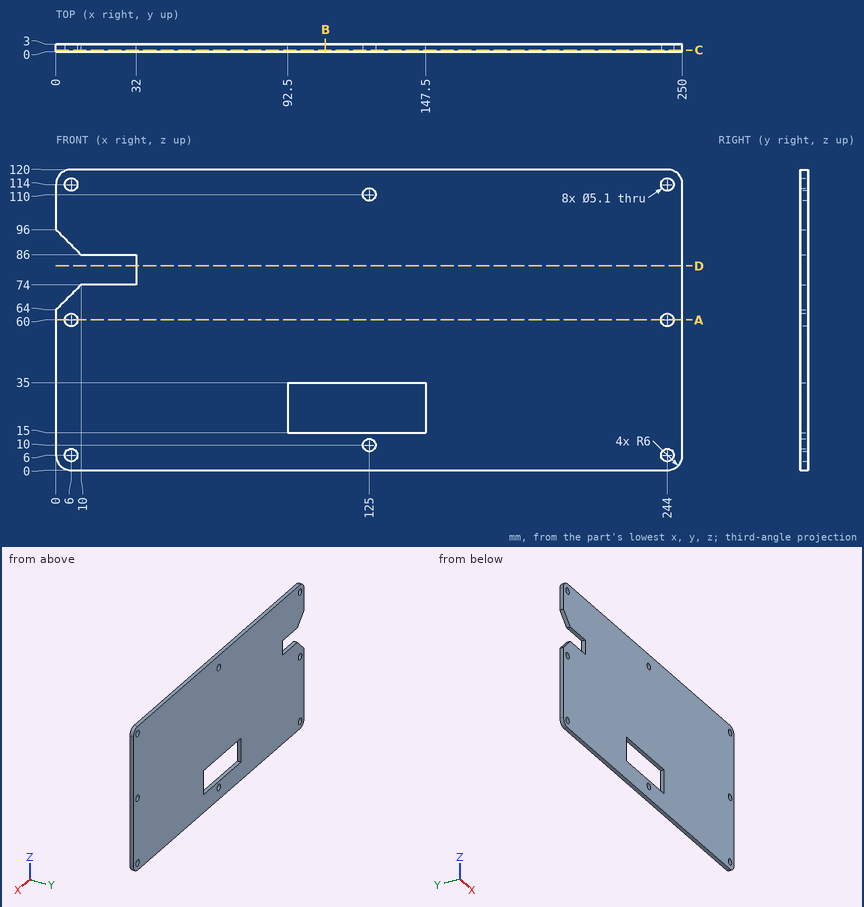
Print and shaded views of the part. All mm, measured from the part's lowest x, y and z. Coordinates: 2 decimals unless noted, no trailing zeros. Write each loop counter-clockwise with the first axis right and the second up, starting at its lowest first coordinate (ties: lowest second). Pieces come first, ordered by that corner, then holes. Notation, with made-up numbers: (56.5, 11.5) -> (115.5, 11.5) arc R25 cw to (115.5, 37.5) -> close; hole circle Ø4 at (37.5, 75). An arc over 180 degrees is marked (long way). Use CSV: the item, a comma, the result in double quotes. Start each with the question number.
Q1. Drill centre lines: probe 1 along Z at (x, y) = (244, 0.7); probe 2 along X at (y, z) = (1.4, 114); probe 3 along X at (y, z) = (2.35, 21). Where is each one in solid material? Low to high.
Q2. Cut at C-C, the plane y = 0.55. State how many separate pieces and enclosed holes the cut face has, then the cut area to 3 significant figures.
Q3. Cut at A-A, the plane z = 60. List the corners of the cut face in (x, y), then the cut area to 3 significant figures.
Q4. Cut at B-B, the plane x = 107.5. List the corners of the cut face in (y, z).
Q5. Cut at D-D, the plane z = 81.5. List the corners of the cut face in (x, y).
Q6. Flat gauge pin, fed straight in: pin 1 Ø1.5 at (x, z) = (103, 34) entering from -Y. Where does the tip first touch, or does it go through?
Checked values:
1,probe 1,"z = 0 to 3.45, 8.55 to 57.45, 62.55 to 111.45, 116.55 to 120"
1,probe 2,"x = 0 to 3.45, 8.55 to 241.45, 246.55 to 250"
1,probe 3,"x = 0 to 92.5, 147.5 to 250"
2,separate pieces,"1"
2,enclosed holes,"9"
2,area,"28,200 mm²"
3,outline,"(0, 0) -> (3.45, 0) -> (3.45, 3) -> (0, 3) -> close; (8.55, 0) -> (241.45, 0) -> (241.45, 3) -> (8.55, 3) -> close; (246.55, 0) -> (250, 0) -> (250, 3) -> (246.55, 3) -> close"
3,area,"719 mm²"
4,outline,"(0, 0) -> (3, 0) -> (3, 15) -> (0, 15) -> close; (0, 35) -> (3, 35) -> (3, 120) -> (0, 120) -> close"
5,outline,"(32, 0) -> (250, 0) -> (250, 3) -> (32, 3) -> close"
6,pin 1,"passes through"
